Design review of the part built by this model. Coordinates are the model's own, in mm. Face numbers are marked on the shaded views. Round coordinates to 2 decimals unless told otherwise and drop trailing zeros. Write each loop counter-clockwise with the first axis right and the second up, starting at its lowest first coordinate (ties: lowest second). Pieces come first, ordered by that corner, then holes.
Autodesk Inventor part; units mm, degrees
ref_plane "YZ Plane" through (0, 0, 0) normal (1, 0, 0) x (0, 1, 0)
ref_plane "XZ Plane" through (0, 0, 0) normal (0, 1, 0) x (-1, 0, 0)
ref_plane "XY Plane" through (0, 0, 0) normal (0, 0, 1) x (1, 0, 0)
sketch "Sketch1" plane through (0, 0, 0) normal (0, 0, 1) x (1, 0, 0)
  arc A0 (-23.5, 0) -> (23.5, 0) centre (0, 0) ccw
  line L0 (30, 0) -> (30, -30)
  line L1 (30, -30) -> (-30, -30)
  line L2 (-30, -30) -> (-30, 0)
  line L3 (-30, 0) -> (-23.5, 0)
  line L4 (23.5, 0) -> (30, 0)
  dimension "d0" = 47
  dimension "d1" = 30
  dimension "d3" = 60
  dimension "d4" = 30
extrude "Extrusion1" add sketch "Sketch1" along normal blind 23
ref_plane "Work Plane1" through (0, 0, 23) normal (0, 0, 1) x (1, 0, 0)
sketch "Sketch2" plane through (0, 0, 23) normal (0, 0, 1) x (1, 0, 0)
  line L0 (30, 0) -> (23.5, 0)
  arc A0 (-23.5, 0) -> (23.5, 0) centre (0, 0) ccw
  arc A1 (-22, 0) -> (22, 0) centre (0, 0) ccw
  line L1 (-23.5, 0) -> (-22, 0)
  line L2 (22, 0) -> (23.5, 0)
  dimension "d8" = 44
extrude "Extrusion2" add sketch "Sketch2" against normal blind 1.5
fillet "Fillet1" radius 2 1 edges at (0, -23.5, 21.5)
ref_plane "Work Plane2" through (0, 0, 0) normal (0, 0, -1) x (-1, 0, 0)
sketch "Sketch3" plane through (0, 0, 0) normal (0, 0, -1) x (-1, 0, 0)
  arc A0 (-23.5, 0) -> (23.5, 0) centre (0, 0) ccw
  arc A1 (-22, 0) -> (22, 0) centre (0, 0) ccw
  line L0 (23.5, 0) -> (30, 0)
  line L1 (23.5, 0) -> (22, 0)
  line L2 (-22, 0) -> (-23.5, 0)
extrude "Extrusion3" add sketch "Sketch3" against normal blind 1.5
fillet "Fillet2" radius 2 1 edges at (0, -23.5, 1.5)
sketch "Sketch4" plane through (-30, 0, 23) normal (0, 1, 0) x (1, 0, 0)
  line L0 (-12, 23) -> (72, 23)
  line L1 (0, 23) -> (0, 0)
  line L2 (53.5, 19.5635) -> (53.5, 3.4365)
  point P0 (30, 23)
  point P1 (3.25, 11.5)
  point P2 (56.75, 11.5)
  dimension "d16" = 11.5
  dimension "d17" = 3.25
  dimension "d18" = 3.25
hole "Hole1" at (-26.75, 0, 11.5) at (26.75, 0, 11.5) direction (0, -1, 0) diameter 3.242 depth 11.8 tip angle 118
sketch "Sketch5" plane through (-30, -30, 0) normal (0, -1, 0) x (1, 0, 0)
  line L0 (0, 0) -> (0, 23)
  line L1 (0, 0) -> (60, 0)
  circle A0 centre (3.25, 11.5) radius 2.5
  circle A1 centre (56.75, 11.5) radius 1.621
  circle A2 centre (56.75, 11.5) radius 2.5
  point P0 (30, 0)
  dimension "d26" = 3.25
  dimension "d27" = 11.5
  dimension "d28" = 5
  dimension "d29" = 5
sketch "Sketch6" plane through (-30, -30, 0) normal (0, -1, 0) x (1, 0, 0)
  line L0 (0, 23) -> (60, 23)
  line L1 (0, 0) -> (60, 0)
  line L2 (0, 23) -> (60, 23)
  line L3 (60, 23) -> (60, 0)
  line L4 (60, 0) -> (0, 0)
  line L5 (0, 0) -> (0, 23)
  point P0 (30, 0)
  point P1 (60, 23)
extrude "Extrusion4" add sketch "Sketch6" along normal blind 27
sketch "Sketch8" plane through (-30, -57, 0) normal (0, -1, 0) x (1, 0, 0)
  line L0 (60, 0) -> (60, 23)
  line L1 (0, 23) -> (0, 0)
  line L2 (60, 23) -> (0, 23)
  point P0 (30, 0)
  point P1 (56.75, 12)
  point P2 (3.25, 12)
  point P3 (60, 11.5)
  point P4 (0, 11.5)
  dimension "d42" = 3.25
  dimension "d43" = 3.25
  dimension "d44" = 11
  dimension "d45" = 11
hole "Hole3" at (26.75, -57, 12) at (-26.75, -57, 12) direction (0, 1, 0) diameter 3.4587 depth 10.8 tip angle 118
equation "\"BendRadius\" = Thickness"
equation "\"BendReliefWidth\" = Thickness"
equation "\"BendReliefDepth\" = 0.5 * Thickness"
equation "\"CornerReliefSize\" = 4 * Thickness"
equation "\"MinimumRemnant\" = 2 * Thickness"
equation "\"TransitionRadius\" = BendRadius"
equation "\"JacobiRadiusSize\" = BendRadius"
equation "\"GapSize\" = Thickness"
properties part number "Bearing housing bottom"
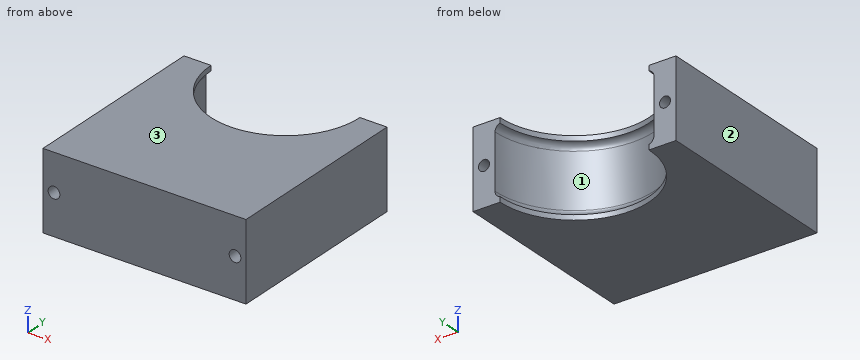
1) Add section A-A on x = 0. State the section outline as (y, z) points, and give its area (3 significant figures).
2) Add section C-C on y = -4.5. Count the separate pieces of the cut face and the enclosed holes in it, and give its area (3 significant figures).
3) Add section D-D on z = 20.5. State the section outline as (x, y) points, and give its area (3 significant figures).
4) The part is to be moulded in two halves that separate along X. For the marked faces 1, 2 and 3, say which applies: pulls with the +X half, pulls with the -X half, needs draft (parallel to the pull), parting line crosses it, or undercut.
5) Add section B-B on z = 5.5. State the section outline as (x, y) points.
6) For line 1 along X through (y, z) = (-54.5, 12); line 2 along X through (y, z) = (-4, 12.5); line 3 along Z through (x, y) = (26.75, -5), list the stretches that pass through material, from the lowest coordinate up.
7) For P1, Ø2, axis at x = -1.5, z = 13.5, coming from the +Y side; P2, Ø1, axis at x = 12.5, z = 10, coming from the +Y side; P3, Ø2.5, axis at x = -26.75, z = 11.5, coming from the +Y side, all flat-tipped, find the tip position at first contact; note any pin that passes through.
Computed:
1. outline: (-57, 0) - (-22, 0) - (-22, 1.5) arc R2 cw to (-23.5, 3.44) - (-23.5, 19.56) arc R2 cw to (-22, 21.5) - (-22, 23) - (-57, 23) - close
1. area: 777 mm2
2. separate pieces: 2
2. enclosed holes: 2
2. area: 315 mm2
3. outline: (-30, -57) - (30, -57) - (30, 0) - (23.27, 0) arc R23.27 cw to (-23.27, 0) - (-30, 0) - close
3. area: 2,570 mm2
4. face 1: undercut
4. face 2: pulls with the -X half
4. face 3: needs draft
5. outline: (-30, -57) - (30, -57) - (30, 0) - (23.5, 0) arc R23.5 cw to (-23.5, 0) - (-30, 0) - close
6. line 1: x = -30 to -28.48, -25.02 to 25.02, 28.48 to 30
6. line 2: x = -30 to -28.03, -25.47 to -23.16, 23.16 to 25.47, 28.03 to 30
6. line 3: z = 0 to 9.88, 13.12 to 23
7. P1: stops at y = -23.37
7. P2: stops at y = -19.58
7. P3: stops at y = -12.02
